Read the model definition and answer for the solid it produces. Units are mm, in the model's axes. Face numbers are marked on the shaded views. A direction names the side the tool comes from. Round coordinates to 2 decimals unless told otherwise and drop trailing zeros. Order: outer loops, then holes, each group sorted by start corner. A loop starts at its lowest first (then second) coordinate and runs counter-clockwise, first axis right, second up. Notation, with made-up numbers: (38.25, 50.5) -> (76.25, 50.5) arc R16 cw to (76.25, 75.5) -> close; hole circle Ø3 at (50.5, 4.5). An arc over 180 degrees is marked (long way). One line per item, written item: value. Start each with the question number.
1. Flat-ended cylindrical pins translate along their axes: pin 1 Ø12 at (x, z) = (-12, 35.5) entering from +Y; pin 2 Ø2 at (x, y) = (30, -64.5) entering from +Z; pin 3 Ø8 at (x, z) = (47, 24.5) entering from +Y. Find the tip coordinate at first contact, or state that the pin passes through.
2. The mould has two halves that part along Y. Classify the marked faces 1, 2 and 3: released by +Y, released by -Y, zero draft, split by the parting line, or undercut.
3. Consider line 1 (X direction, y = 0, z = 25); line 2 (X direction, y = -31, z = 17); line 3 (Y direction, x = -27, z = 23). Determine where each line is inside the solid, lowest interval first.
4. Section A-A (z = 44.5) is taken. Give the vertices of the cut face in (x, y).
5. For the marked faces 4, 5 and 6, determine the directions among +Z, -Z, +X, -X, +Y, -Y from which every point of the face is accessible in a straight line to the end or side of a thin tool.
from build123d import *

# Parameters (mm, degrees)
F2_T = 2.54
F3_R = 5.08


# Not quite as in the source:
# - a shell that OpenCascade refuses in one call is made with other operations: the cavity is built on its own and cut out


with BuildPart() as f1:
    # F0 (on Front) → F1 (revolve)
    with BuildSketch(Plane.XZ):
        with BuildLine():
            ThreePointArc((-57.9764892951, 60.004751325), (-62.3916472883, 58.1048437598), (-64.2108023167, 53.6558052296))
            Line((-64.2108023167, 53.6558052296), (-64.2108023167, 9.8601095378))
            Line((-64.2108023167, 9.8601095378), (-14.9272382259, 9.8601095378))
            Line((-14.9272382259, 9.8601095378), (-14.9272382259, 32.7742578626))
            ThreePointArc((-14.9272382259, 32.7742578626), (-13.0673662865, 37.2643859231), (-8.5772382259, 39.1242578626))
            Line((-8.5772382259, 39.1242578626), (24.8787216842, 39.1242578626))
            Line((24.8787216842, 39.1242578626), (24.8787216842, 61.514493078))
            Line((24.8787216842, 61.514493078), (-57.9764892951, 60.004751325))
        make_face()
    revolve(axis=Axis((24.8787216842, 0, 50.3193754703), (0, 0, 1)))

    # F2: shell of thickness 2.54, made by hand


with BuildPart() as f2_core1:
    # F2_t2: copy of F1
    add(f1.part)

    # the walls: a layer under each face that stays
    f2_faces = [f2_core1.faces().sort_by_distance(p)[0] for p in [
        (112.1490906567, 0, 58.1048437598),
        (113.9682456851, 0, 31.7579573837),
        (84.2717376848, 59.3930160006, 9.8601095378),
        (64.6846815944, 0, 21.3171837002),
        (62.8248096549, 0, 37.2643859231),
        (24.8787216842, 0, 39.1242578626),
    ]]
    thicken(f2_faces, amount=-F2_T, mode=Mode.SUBTRACT)


with BuildPart() as f1_1:
    add(f1.part)

    # what is left inside the walls is the cavity
    f2_cavity = [f2_core1.part.solids().sort_by_distance(p)[0] for p in [
        (111.402846, 0, 39.903907),
    ]]
    add(f2_cavity, mode=Mode.SUBTRACT)

    # F3
    f3_edges = [f1_1.edges().sort_by_distance(p)[0] for p in [
        (64.684682, 0, 9.86011),
    ]]
    fillet(f3_edges, radius=F3_R)


solid = f1_1.part
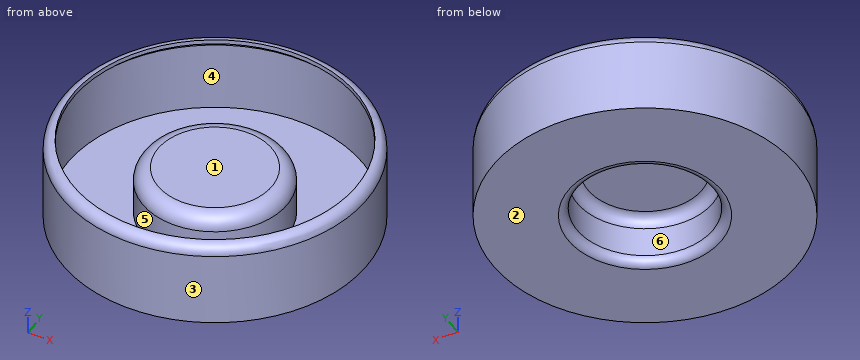
Answer:
1. pin 1: y = 83.57
1. pin 2: z = 12.4
1. pin 3: y = 87.23
2. face 1: undercut
2. face 2: zero draft
2. face 3: split by the parting line
3. line 1: -64.21 to -61.67, -17.47 to -14.93, 64.68 to 67.22, 111.43 to 113.97
3. line 2: -58.64 to -55.93, -3.97 to -0.09, 49.85 to 53.73, 105.69 to 108.4
3. line 3: -72.43 to -69.28, 69.28 to 72.43
4. outline: circle Ø178.18 at (24.88, 0); hole circle Ø173.1 at (24.88, 0)
5. face 4: none
5. face 5: +Z
5. face 6: -Z
